Part print with two shaded views. Sizes in mm from the minimum x, y, z corner. Coordinates: 2 decimals unless noted, no trailing zeros. Write each loop counter-clockwise with the first axis right and the second up, starting at its lowest first coordinate (ties: lowest second). Pieces come first, ordered by that corner, then holes. Notation, with made-up numbers: (2, -17) - (41, -17) arc R14 ccw to (41, -2) - close; hole circle Ø8 at (-9.5, -2.5). An arc over 180 degrees is marked (long way). Answer in a Markdown table with one row per item. Add a question column.
Q1. Band-saw the part on A-A (z = 3.35). List the corners of the cut face in (x, y), and give its area (3 significant figures).
Q2. Drill centre lines: line 1 along X through (y, z) = (2.4, 3.35); line 2 along Z through (x, y) = (10, 3.65); line 3 along X through (y, z) = (1, 56). Where is each one in solid material? Low to high. Write a range as from..to.
Q3. Band-saw the part on B-B (x = 28.95). List the corners of the cut face in (y, z), and give its area (3 significant figures).
Q4. Band-saw the part on C-C (y = 2). List the corners of the cut face in (x, z), and give its area (3 significant figures).
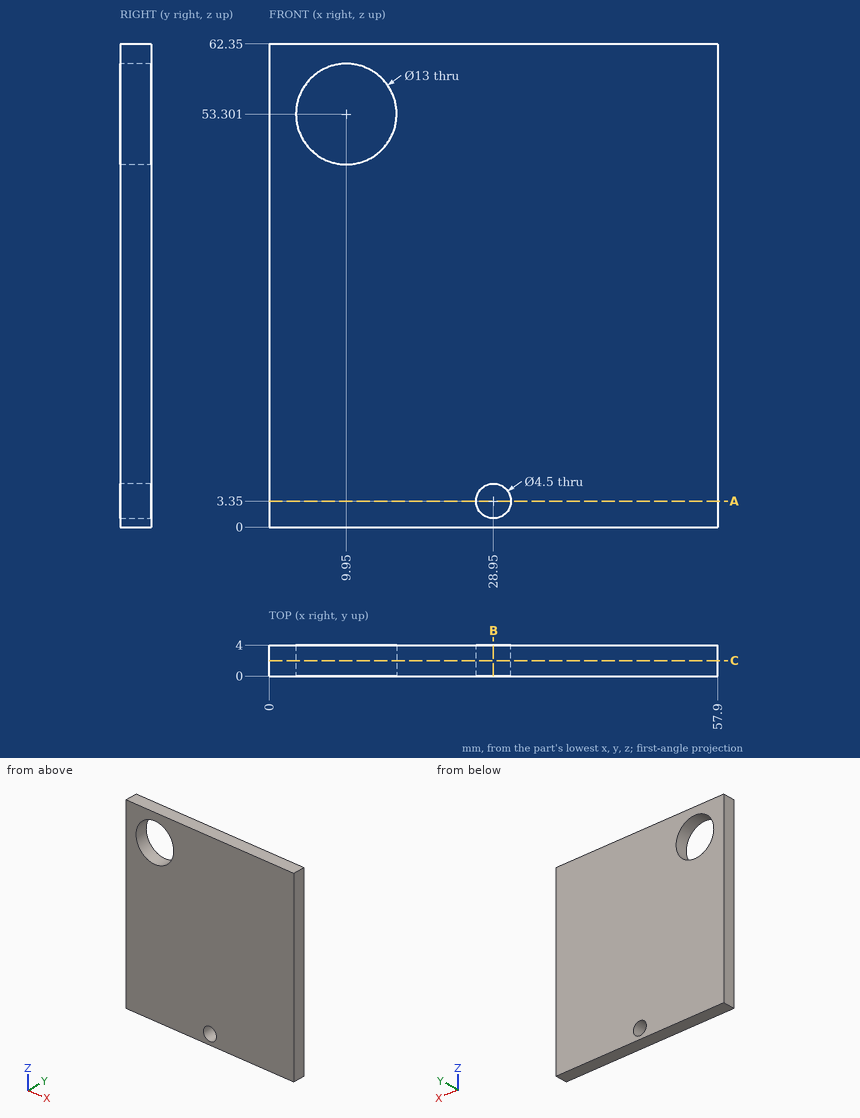
Checked values:
| question | item | result |
|---|---|---|
| 1 | outline | (0, 0) - (26.7, 0) - (26.7, 4) - (0, 4) - close; (31.2, 0) - (57.9, 0) - (57.9, 4) - (31.2, 4) - close |
| 1 | area | 214 mm² |
| 2 | line 1 | x = 0..26.7, 31.2..57.9 |
| 2 | line 2 | z = 0..46.8, 59.8..62.35 |
| 2 | line 3 | x = 0..4.04, 15.86..57.9 |
| 3 | outline | (0, 0) - (4, 0) - (4, 1.1) - (0, 1.1) - close; (0, 5.6) - (4, 5.6) - (4, 62.35) - (0, 62.35) - close |
| 3 | area | 231 mm² |
| 4 | outline | (0, 0) - (57.9, 0) - (57.9, 62.35) - (0, 62.35) - close; hole circle Ø13 at (9.95, 53.3); hole circle Ø4.5 at (28.95, 3.35) |
| 4 | area | 3,460 mm² |
